Work out the finished part from the listing and answer in its coordinate system (mm). Round coordinates to 2 decimals unless told otherwise and drop trailing zeros. Order: outer loops, then holes, each group sorted by start corner. A loop starts at its lowest first (then second) coordinate and runs counter-clockwise, first axis right, second up. Notation, with made-up numbers: (30, -21) -> (71, -21) arc R28 ccw to (71, 1) -> close; hole circle Ø5 at (5, -4.75). An arc over 180 degrees is marked (long way). Use a Markdown table: item, result. Add a question column.
Item 1: A cutting plane is placed at B-B, the plane y = -15. Determine the outline of the cut face in (x, z).
Item 2: Find the intervals of material crossed by L1, parallel to Z at x = -5.75, y = 21; L2, parallel to Z at x = -0.25, y = 0, in increasing order. Write a range as [from, to].
Item 3: Flat-ended cylindrical pins translate along their axes: P1, Ø1.5, axis at y = 5, z = 2, coming from the +X side; P2, Ø4, axis at y = -33.5, z = -4.5, coming from the -X side; P3, Ø8, axis at x = -6, y = -16.5, coming from the +Z side. Find the tip coordinate at first contact, or state that the pin passes through.
Item 4: A cutting plane is placed at A-A, the plane y = 8.5. Determine the outline of the cut face in (x, z), plus the area to 3 significant figures.
from build123d import *

# Parameters (mm, degrees)
SKETCH_608_R    = 8
EXTRUDE_1_DEPTH = 25


# Read off the part's stored shape, not the designer's step: 凸台-拉伸2
with BuildPart() as part:
    # Sketch 608 → 凸台-拉伸1 (new body)
    with BuildSketch(Plane(origin=(0, 0, 0), x_dir=(1, 0, 0), z_dir=(0, 1, 0))):
        with Locations(Location((0, 0, 0), (0, 0, 270))):
            Circle(SKETCH_608_R)
    extrude(amount=EXTRUDE_1_DEPTH)

    # 凸台-拉伸2 outline → 凸台-拉伸2 (revolve)
    with BuildSketch(Plane.XY):
        Polygon((0, -24), (6.742213297, -24), (8, 0), (0, 0), align=None)
    revolve(axis=Axis((0, 0, 0), (0, 1, 0)))

    # 草图7 → 旋转4 (revolve)
    with BuildSketch(Plane.XY, mode=Mode.PRIVATE) as revolve_4_sk:
        with BuildLine():
            Line((0, -24), (6.742213297, -24))
            Line((6.742213297, -24), (5.571871993, -40.736660394))
            ThreePointArc((5.571871993, -40.736660394), (4.125623062, -43.768784333), (1, -45))
            Line((1, -45), (0, -45))
            Line((0, -45), (0, -24))
        make_face()
    revolve(revolve_4_sk.sketch.rotate(Axis((0, -24, 0), (0, -1, 0)), 180), axis=Axis((0, -24, 0), (0, -1, 0)))


solid = part.part
Reported:
| question | item | result |
|---|---|---|
| 1 | outline | circle Ø14.43 at (0, 0) |
| 2 | L1 | [-5.56, 5.56] |
| 2 | L2 | [-8, 8] |
| 3 | P1 | x = 7.9 |
| 3 | P2 | x = -5.55 |
| 3 | P3 | z = 6.87 |
| 4 | outline | circle Ø16 at (0, 0) |
| 4 | area | 201 mm² |
